from build123d import *

# Parameters (mm, degrees)
SKETCH1_W           = 50
SKETCH1_H           = 50
BOSS_EXTRUDE3_DEPTH = 8
SKETCH6_R           = 3.8
CUT_EXTRUDE2_DEPTH  = 68


with BuildPart() as part:
    # Sketch1 → Boss-Extrude3 (new body)
    with BuildSketch(Plane.XY):
        with Locations((25, 25)):
            Rectangle(SKETCH1_W, SKETCH1_H)
    extrude(amount=BOSS_EXTRUDE3_DEPTH)

    # Sketch6 → Cut-Extrude2 (cut)
    with BuildSketch(Plane.XZ):
        with Locations((0, 4)):
            Circle(SKETCH6_R)
        with Locations((50, 4)):
            Circle(SKETCH6_R)
    extrude(amount=-CUT_EXTRUDE2_DEPTH, mode=Mode.SUBTRACT)


solid = part.part
Could you check a few things on this model? Use its own coordinates, in mm. Round coordinates to 2 decimals unless told otherwise and drop trailing zeros. Write each loop counter-clockwise with the first axis right and the second up, starting at its lowest first coordinate (ties: lowest second). Pieces come first, ordered by that corner, then holes. Notation, with made-up numbers: (-17, 33.25) - (-5, 33.25) arc R28 ccw to (-5, 67.25) - close; hole circle Ø9 at (53.5, 58.25). An arc over 180 degrees is marked (long way). Use a Markdown table: item, result.
Q1. I want a section at B-B (z = 4). List the corners of the cut face in (x, y) for me.
Output values:
| item | result |
|---|---|
| outline | (3.8, 0) - (46.2, 0) - (46.2, 50) - (3.8, 50) - close |
Q2. Please list where these lines run through material, in increasing order: L1, parallel to Z at x = 48.5, y = 3; L2, parallel to X at y = 10, z = 4.75; L3, parallel to X at y = 37.5, z = 0.5.
Output values:
| item | result |
|---|---|
| L1 | 0 to 0.51, 7.49 to 8 |
| L2 | 3.73 to 46.27 |
| L3 | 1.48 to 48.52 |
Q3. Thinking about a two-plate mould opening in Z: for faces 1 (the cylindrical face through (3.8, 24.6, 3.9)), 2 (the flat face through (25, 50, 4)), 3 (the flat face through (25, 25, 8)), which applies, released by +Z, released by -Z, zero draft, split by the parting line, or undercut?
Output values:
| item | result |
|---|---|
| face 1 | undercut |
| face 2 | zero draft |
| face 3 | released by +Z |
Q4. I want a section at C-C (z = 6.5). List the corners of the cut face in (x, y) for me, plus the area to 3 significant figures.
Output values:
| item | result |
|---|---|
| outline | (2.86, 0) - (47.14, 0) - (47.14, 50) - (2.86, 50) - close |
| area | 2,210 mm2 |
Q5. I want a section at A-A (y = 18). List the corners of the cut face in (x, z) for me.
Output values:
| item | result |
|---|---|
| outline | (0, 0) - (50, 0) - (50, 0.2) arc R3.8 cw to (50, 7.8) - (50, 8) - (0, 8) - (0, 7.8) arc R3.8 cw to (0, 0.2) - close |
